Part model, mm, in its own coordinate system. Face numbers are marked on the shaded views. Round coordinates to 2 decimals unless told otherwise and drop trailing zeros. Order: outer loops, then holes, each group sorted by start corner. A loop starts at its lowest first (then second) coordinate and runs counter-clockwise, first axis right, second up. Notation, with made-up numbers: (-21, 85.5) -> (29, 85.5) arc R27 cw to (29, 114.5) -> close; hole circle Ø10 at (26.25, -5). An arc over 180 degrees is marked (long way). Use CSV: the item, a comma, the result in double quotes.
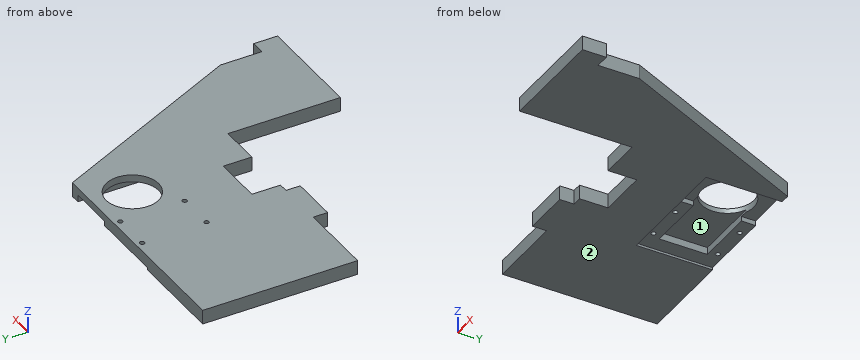
```python
from build123d import *

# Parameters (mm, degrees)
ESQUISSE1_W             = 135
ESQUISSE1_H             = 112.17
BOSS_EXTRU_1_DEPTH      = 6
ENL_V_MAT_EXTRU_1_DEPTH = 6
ESQUISSE3_W             = 6
ESQUISSE3_H             = 10
ESQUISSE3_W_2           = 20
ESQUISSE3_H_2           = 6
BOSS_EXTRU_2_DEPTH      = 6
ESQUISSE4_W             = 51
ESQUISSE4_H             = 32
ENL_V_MAT_EXTRU_5_DEPTH = 3
ESQUISSE7_R             = 11
ENL_V_MAT_EXTRU_6_DEPTH = 4
ESQUISSE8_W             = 30
ESQUISSE8_H             = 20.2
ENL_V_MAT_EXTRU_7_DEPTH = 1
ESQUISSE9_W             = 25
ESQUISSE9_H             = 5.9
BOSS_EXTRU_4_DEPTH      = 2
ESQUISSE10_W            = 25
ESQUISSE10_H            = 5.9
BOSS_EXTRU_5_DEPTH      = 2
ESQUISSE11_W            = 6.5
ESQUISSE11_H            = 32
BOSS_EXTRU_6_DEPTH      = 2
ESQUISSE12_R            = 1
ENL_V_MAT_EXTRU_8_DEPTH = 6
ESQUISSE13_W            = 21
ESQUISSE13_H            = 12
ENL_V_MAT_EXTRU_9_DEPTH = 6


with BuildPart() as part:
    # Esquisse1 → Boss.-Extru.1 (new body)
    with BuildSketch(Plane.XY):
        Rectangle(ESQUISSE1_W, ESQUISSE1_H)
    extrude(amount=BOSS_EXTRU_1_DEPTH)

    # Esquisse2 → Enlèv. mat.-Extru.1 (cut)
    with BuildSketch(Plane.XY.offset(6)):
        Polygon((27.5, -56.085), (-67.5, -56.085), (-67.5, -8.915), (-38.5, -8.915), (27.5, -8.915), align=None)
        Polygon((67.5, -28.665), (27.980425971, 56.085), (67.5, 56.085), align=None)
    extrude(amount=-ENL_V_MAT_EXTRU_1_DEPTH, mode=Mode.SUBTRACT)

    # Esquisse3 → Boss.-Extru.2 (add)
    with BuildSketch(Plane.XY.offset(6)):
        with Locations((70.5, -51.085)):
            Rectangle(ESQUISSE3_W, ESQUISSE3_H)
        with Locations((-25, -11.915)):
            Rectangle(ESQUISSE3_W_2, ESQUISSE3_H_2)
    extrude(amount=-BOSS_EXTRU_2_DEPTH)

    # Esquisse4 → Enlèv. mat.-Extru.5 (cut)
    with BuildSketch(Plane(origin=(0, 0, 0), x_dir=(-1, 0, 0), z_dir=(0, 0, -1))):
        with Locations((1.519574029, 40.085)):
            Rectangle(ESQUISSE4_W, ESQUISSE4_H)
    extrude(amount=-ENL_V_MAT_EXTRU_5_DEPTH, mode=Mode.SUBTRACT)

    # Esquisse7 → Enlèv. mat.-Extru.6 (cut, through all)
    with BuildSketch(Plane(origin=(0, 0, 3), x_dir=(-1, 0, 0), z_dir=(0, 0, -1))):
        with Locations((-11.980425971, 40.085)):
            Circle(ESQUISSE7_R)
    extrude(amount=-ENL_V_MAT_EXTRU_6_DEPTH, mode=Mode.SUBTRACT)

    # Esquisse8 → Enlèv. mat.-Extru.7 (cut)
    with BuildSketch(Plane(origin=(0, 0, 3), x_dir=(-1, 0, 0), z_dir=(0, 0, -1))):
        with Locations((5.519574029, 40.085)):
            Rectangle(ESQUISSE8_W, ESQUISSE8_H)
    extrude(amount=-ENL_V_MAT_EXTRU_7_DEPTH, mode=Mode.SUBTRACT)

    # Esquisse9 → Boss.-Extru.4 (add)
    with BuildSketch(Plane(origin=(0, 0, 3), x_dir=(-1, 0, 0), z_dir=(0, 0, -1))):
        with Locations((8.019574029, 53.135)):
            Rectangle(ESQUISSE9_W, ESQUISSE9_H)
    extrude(amount=BOSS_EXTRU_4_DEPTH)

    # Esquisse10 → Boss.-Extru.5 (add)
    with BuildSketch(Plane(origin=(0, 0, 3), x_dir=(-1, 0, 0), z_dir=(0, 0, -1))):
        with Locations((8.019574029, 27.035)):
            Rectangle(ESQUISSE10_W, ESQUISSE10_H)
    extrude(amount=BOSS_EXTRU_5_DEPTH)

    # Esquisse11 → Boss.-Extru.6 (add)
    with BuildSketch(Plane(origin=(0, 0, 3), x_dir=(-1, 0, 0), z_dir=(0, 0, -1))):
        with Locations((23.769574029, 40.085)):
            Rectangle(ESQUISSE11_W, ESQUISSE11_H)
    extrude(amount=BOSS_EXTRU_6_DEPTH)

    # Esquisse12 → Enlèv. mat.-Extru.8 (cut, through all)
    with BuildSketch(Plane(origin=(0, 0, 1), x_dir=(-1, 0, 0), z_dir=(0, 0, -1))):
        with Locations((2.519574029, 53.435)):
            Circle(ESQUISSE12_R)
        with Locations((18.519574029, 53.435)):
            Circle(ESQUISSE12_R)
        with Locations((2.519574029, 26.435)):
            Circle(ESQUISSE12_R)
        with Locations((18.519574029, 26.435)):
            Circle(ESQUISSE12_R)
    extrude(amount=-ENL_V_MAT_EXTRU_8_DEPTH, mode=Mode.SUBTRACT)

    # Esquisse13 → Enlèv. mat.-Extru.9 (cut)
    with BuildSketch(Plane.XY.offset(6)):
        with Locations((-0.5, -2.915)):
            Rectangle(ESQUISSE13_W, ESQUISSE13_H)
    extrude(amount=-ENL_V_MAT_EXTRU_9_DEPTH, mode=Mode.SUBTRACT)


solid = part.part
```
(1) Drop flat-ended pins along their axis: P1, Ø1, axis at y = -42, z = 4, coming from the +X side; P2, Ø1, axis at x = 0, y = 32.5, coming from the -Z side; P3, Ø3, axis at x = 72, z = 4.5, coming from the +Y side (3 decimals); P4, Ø1, axis at x = -20.5, y = -16.5, coming from the -Z side. Give the stop position or say it passes through.
Reply:
P1,"x = 67.5"
P2,"z = 4"
P3,"y = -46.085"
P4,"through"
(2) Cut at B-B, the plane y = 35.5. Give the cut face in (x, z).
Reply:
outline,"(-67.5, 0) -> (-27.02, 0) -> (-27.02, 1) -> (-20.52, 1) -> (-20.52, 4) -> (1.98, 4) -> (1.98, 6) -> (-67.5, 6) -> close; (21.98, 3) -> (23.98, 3) -> (23.98, 0) -> (37.58, 0) -> (37.58, 6) -> (21.98, 6) -> close"
(3) Cut at A-A, the plane x = -12.5. Give the cut face in (y, z) (3 decimals).
Reply:
outline,"(-8.915, 0) -> (24.085, 0) -> (24.085, 1) -> (29.985, 1) -> (29.985, 4) -> (50.185, 4) -> (50.185, 1) -> (56.085, 1) -> (56.085, 6) -> (-8.915, 6) -> close"
(4) Cut at D-D, the plane y = -3. Give the cut face in (x, z).
Reply:
outline,"(-67.5, 0) -> (-11, 0) -> (-11, 6) -> (-67.5, 6) -> close; (10, 0) -> (55.53, 0) -> (55.53, 6) -> (10, 6) -> close"
(5) Pull direction Y, two halves, no side cores. Call the marked faces 1 and 2: released by +Y, released by -Y, zero draft, split by the parting line, or undercut.
Reply:
face 1,"undercut"
face 2,"zero draft"
(6) Probe probe 1 along Y at (x, z) = (-12, 2.7) (3 decimals); probe 2 along Y at (x, z) = (11.5, 5.75) (1 decimal); probe 3 along X at (y, z) = (-38, 4.6). List the from-to ranges inside material, lowest first. Write a range as [from, to].
Reply:
probe 1,"[-8.915, 29.985], [50.185, 56.085]"
probe 2,"[-8.9, 29.1], [51.1, 56.1]"
probe 3,"[27.5, 67.5]"
(7) Cut at C-C, the plane x = 19. Give the cut face in (y, z) (3 decimals), then the cut area to 3 significant figures.
Reply:
outline,"(-8.915, 0) -> (24.085, 0) -> (24.085, 3) -> (31.616, 3) -> (31.616, 6) -> (-8.915, 6) -> close; (48.554, 3) -> (56.085, 3) -> (56.085, 6) -> (48.554, 6) -> close"
area,"243 mm2"
